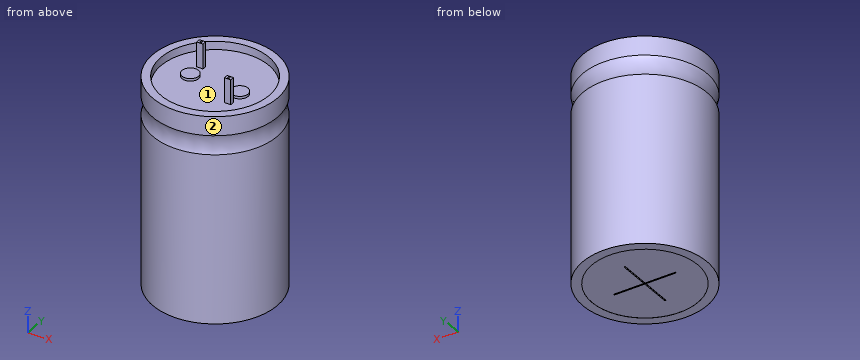
Autodesk Inventor part; units mm, degrees
ref_plane "Arbeitsebene1" through (-6, 4, 54.001) normal (0.5547, 0.8321, 0) x (0, 0, 1)
ref_plane "YZ Plane" through (0, 0, 0) normal (1, 0, 0) x (0, 1, 0)
ref_plane "XZ Plane" through (0, 0, 0) normal (0, 1, 0) x (-1, 0, 0)
sketch "Skizze1" plane through (0, 0, 0) normal (0, 1, 0) x (-1, 0, 0)
  line L0 (0, 0) -> (0, 50)
  line L1 (0, 50) -> (-15, 50)
  line L2 (-15, 50) -> (-15, 45.4)
  line L3 (-15, 40.8) -> (-15, 0)
  arc A0 (-15, 40.8) -> (-15, 45.4) centre (-20.6528, 43.1) ccw
  line L4 (0, 0) -> (-15, 0)
  line L5 (0, -10) -> (0, 60)
  dimension "d0" = 50
  dimension "d1" = 15
  dimension "d2" = 4.6
  dimension "d72" = 14.55
  dimension "d73" = 4.6
revolve "Umdrehung1" add sketch "Skizze1" angle 360 about axis through (0, 0, -10) along (0, 0, 1)
sketch "Skizze3" plane through (0, 0, 50) normal (0, 0, 1) x (1, 0, 0)
  circle A0 centre (0, 0) radius 13.05
  dimension "d10" = 26.1
extrude "Extrusion2" cut sketch "Skizze3" against normal blind 2
sketch "Skizze7" plane through (0, 0, 0) normal (0, 0, -1) x (-1, 0, 0)
  circle A0 centre (0, 0) radius 12.8
  dimension "d19" = 25.6
extrude "Extrusion4" cut sketch "Skizze7" against normal blind 0.02
sketch "Skizze17" plane through (0, 0, 48) normal (0, 0, 1) x (1, 0, 0)
  line L0 (-4.2414, 0) -> (6, 0) construction
  line L1 (6, 0) -> (-6, 0) construction
  line L2 (6, 0) -> (6, -3.5) construction
  line L3 (-6, 0) -> (-6, 3.5) construction
  line L4 (-6, 3.5) -> (6, -3.5) construction
  circle A0 centre (-6, 0) radius 2
  circle A1 centre (6, 0) radius 2
  line L5 (-6.75, 4.5) -> (-5.25, 4.5)
  line L6 (-5.25, 4.5) -> (-5.25, 3.5)
  line L7 (-5.25, 3.5) -> (-6.75, 3.5)
  line L8 (-6.75, 3.5) -> (-6.75, 4.5)
  line L9 (6.75, -3.5) -> (5.25, -3.5)
  line L10 (5.25, -3.5) -> (5.25, -4.5)
  line L11 (5.25, -4.5) -> (6.75, -4.5)
  line L12 (6.75, -4.5) -> (6.75, -3.5)
  point P0 (0, 0)
  point P1 (0, 0)
  dimension "d54" = 12
  dimension "d55" = 3.5
  dimension "d56" = 3.5
  dimension "d57" = 4
  dimension "d58" = 4
  dimension "d59" = 1.5
  dimension "d60" = 1
  dimension "d61" = 1.5
  dimension "d62" = 1
extrude "Extrusion8" add sketch "Skizze17" along normal blind 0.6 contours A0 | A1
sketch "Skizze18" plane through (0, 0, 48) normal (0, 0, 1) x (1, 0, 0)
  line L0 (-6.75, 4.5) -> (-5.25, 4.5)
  line L1 (-5.25, 4.5) -> (-5.25, 3.5)
  line L2 (-5.25, 3.5) -> (-6.75, 3.5)
  line L3 (-6.75, 3.5) -> (-6.75, 4.5)
  line L4 (6.75, -3.5) -> (5.25, -3.5)
  line L5 (5.25, -3.5) -> (5.25, -4.5)
  line L6 (5.25, -4.5) -> (6.75, -4.5)
  line L7 (6.75, -4.5) -> (6.75, -3.5)
  point P0 (0, 0)
  point P1 (-6, 3.5)
  point P2 (6, -3.5)
  dimension "d66" = 1.5
  dimension "d67" = 1
  dimension "d68" = 1.5
  dimension "d69" = 1
extrude "Extrusion9" add sketch "Skizze18" along normal blind 6
sketch "Skizze9" plane through (0, 0, 0.02) normal (0, 0, -1) x (-1, 0, 0)
  line L0 (-7.5, 0) -> (7.5, 0) construction
  line L1 (0, 4.0384) -> (0, 7.5) construction
  line L2 (0, 7.5) -> (0, -7.5) construction
  line L3 (0.15, 7.5) -> (-0.15, 7.5)
  line L4 (-0.15, 7.5) -> (-0.15, 0.15)
  line L5 (-0.15, 0.15) -> (-7.5, 0.15)
  line L6 (-7.5, 0.15) -> (-7.5, -0.15)
  line L7 (-7.5, -0.15) -> (-0.15, -0.15)
  line L8 (-0.15, -0.15) -> (-0.15, -7.5)
  line L9 (-0.15, -7.5) -> (0.15, -7.5)
  line L10 (0.15, -7.5) -> (0.15, -0.15)
  line L11 (0.15, -0.15) -> (7.5, -0.15)
  line L12 (7.5, -0.15) -> (7.5, 0.15)
  line L13 (7.5, 0.15) -> (0.15, 0.15)
  line L14 (0.15, 0.15) -> (0.15, 7.5)
  point P0 (0, 0)
  point P1 (0, 0)
  dimension "d23" = 15
  dimension "d24" = 15
  dimension "d74" = 0.3
extrude "Extrusion10" cut sketch "Skizze9" against normal blind 0.3
sketch "Skizze19" plane through (0, 0, 54) normal (0, 0, 1) x (1, 0, 0)
  line L0 (6.75, -3.5) -> (5.25, -3.5)
  line L1 (6.75, -3.5) -> (5.25, -3.5)
  line L2 (5.25, -3.5) -> (5.25, -4.5)
  line L3 (5.25, -4.5) -> (6.75, -4.5)
  line L4 (6.75, -4.5) -> (6.75, -3.5)
  line L5 (5.25, -3.5) -> (6.75, -4.5) construction
  circle A0 centre (6, -4) radius 0.25
  line L6 (-5.25, 3.5) -> (-5.25, 4.5)
  line L7 (-5.25, 4.5) -> (-6.75, 4.5)
  line L8 (-6.75, 4.5) -> (-6.75, 3.5)
  line L9 (-6.75, 3.5) -> (-5.25, 3.5)
  line L10 (-5.25, 4.5) -> (-6.75, 4.5) construction
  line L11 (-6.75, 4.5) -> (-5.25, 3.5) construction
  circle A1 centre (-6, 4) radius 0.25
  point P0 (0, 0)
  dimension "d77" = 0.5
  dimension "d78" = 0.5
extrude "Extrusion11" add sketch "Skizze19" along normal blind 0.001 contours A0 | A1
ref_plane "Arbeitsebene1" through (-6, 4, 54.001) normal (0.5547, 0.8321, 0) x (0, 0, 1)
properties part number "capacitor (LGN2X151MELB50)"
Check sheet for the modelled part. Datum: model origin and axes. Units: mm. Face numbers are marked on the shaded views. Coordinates: 2 decimals unless noted, no trailing zeros. Order: outer loops, then holes, each group sorted by start corner. A loop starts at its lowest first (then second) coordinate and runs counter-clockwise, first axis right, second up. Notation, with made-up numbers: M 6,35.5 L 18,35.5 A28 cw 18,58.5 Z; hole C 43,67 d3. An arc over 180 degrees is marked long. One line per question, with ' | ' between items. Start each with the question number.
Item 1: Sectioned sample at A-A on z = 8. Record the cut outline in (x, y), and give its area (3 significant figures).
Item 2: Material ranges on line 1 (Y direction, x = 0, z = 49); line 2 (Z direction, x = -11, y = 2); line 3 (Y direction, x = 3.5, z = 10.5), recorded low to high.
Item 3: Gauge pin test, flat ends, axial feed: P1, Ø0.8, axis at x = 6.5, z = 52, coming from the -Y side; P2, Ø2, axis at x = 12, y = 5, coming from the +Z side; P3, Ø4.5, axis at x = -6.5, y = 0.5, coming from the +Z side. Record the tip position at first contact, or that the pin passes through.
Item 4: Mould release check, pull along Y, two halves, no side actions. Record for the marked faces 1 and 2: pulls with the +Y half, pulls with the -Y half, needs draft (parallel to the pull), parting line crosses it, or undercut.
Answer below:
1) outline: C 0,0 d30 | area: 707 mm^2
2) line 1: y = -15 to -13.05, 13.05 to 15 | line 2: z = 0.02 to 48 | line 3: y = -14.59 to 14.59
3) P1: stops at y = -4.5 | P2: stops at z = 50 | P3: stops at z = 48.6
4) face 1: undercut | face 2: parting line crosses it
